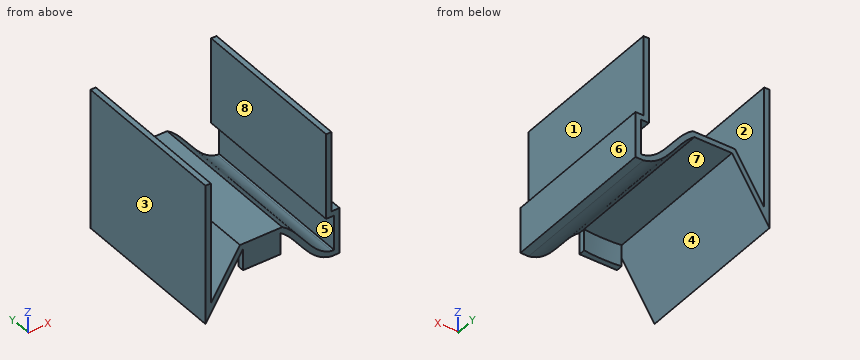
from build123d import *

# Parameters (mm, degrees)
BOSS_EXTRUDE12_DEPTH = 60
BOSS_EXTRUDE13_DEPTH = 8


with BuildPart() as part:
    # Sketch1 → Boss-Extrude12 (new body)
    with BuildSketch(Plane(origin=(0, 0, 0), x_dir=(1, 0, 0), z_dir=(0, 1, 0))):
        with BuildLine():
            Line((3, 47), (3, 30))
            Line((3, 30), (0, 30))
            Line((0, 30), (0, 0))
            Line((0, 0), (-2, 0))
            Line((-2, 0), (-2, 32))
            Line((-2, 32), (1, 32))
            Line((1, 32), (1, 45))
            Line((1, 45), (0.176102142, 45))
            add(Edge.make_bspline(
                [(-18.386432119, 28), (-18.281589374, 28.071011485), (-18.076006872, 28.210643772), (-17.632017964, 28.509033814), (-16.788752159, 29.127765228), (-15.266101597, 30.436706514), (-13.281769764, 32.578807621), (-11.116323446, 35.322397153), (-8.327983452, 38.971629637), (-4.796332276, 42.989291988), (-1.605396872, 44.667429051), (0.176102142, 45)],
                knots=[0.007315744, 0.007315744, 0.007315744, 0.007315744, 0.023228008, 0.039140272, 0.0709648, 0.134613856, 0.261911967, 0.389210078, 0.516508189, 0.771104411, 1.025700634, 1.025700634, 1.025700634, 1.025700634], degree=3))
            Line((-18.386432119, 28), (-34.105031298, 28))
            Line((-34.105031298, 28), (-45, 45.32952773))
            Line((-45, 45.32952773), (-45, 0))
            Line((-45, 0), (-47, 0))
            Line((-47, 0), (-47, 52.268387809))
            Line((-47, 52.268387809), (-33, 30))
            Line((-33, 30), (-19, 30))
            add(Edge.make_bspline(
                [(0, 47), (-8.735842334, 45.522262704), (-12.411198706, 34.462689008), (-19, 30)],
                knots=[0, 0, 0, 0, 1, 1, 1, 1], degree=3))
            Line((0, 47), (3, 47))
        make_face()
    extrude(amount=BOSS_EXTRUDE12_DEPTH)

    # Sketch2 → Boss-Extrude13 (add)
    with BuildSketch(Plane(origin=(0, 0, -30), x_dir=(-1, 0, 0), z_dir=(0, 0, -1))):
        with BuildLine():
            Line((33, 0), (19, 0))
            Line((19, 0), (19, 2.423963318))
            ThreePointArc((19, 2.423963318), (26, 2), (33, 2.423963318))
            Line((33, 2.423963318), (33, 0))
        make_face()
    extrude(amount=BOSS_EXTRUDE13_DEPTH)


solid = part.part
Check sheet for the modelled part. Datum: model origin and axes. Units: mm. Face numbers are marked on the shaded views. A direction names the side the tool comes from. Round coordinates to 2 decimals unless told otherwise and drop trailing zeros. Order: outer loops, then holes, each group sorted by start corner. A loop starts at its lowest first (then second) coordinate and runs counter-clockwise, first axis right, second up.
Q1. Cross-section at C-C, the plane x = -21.5. Enter the section's corners in (y, z), plus the area to 3 significant figures.
Filled sheet:
outline: (0, -38) - (2.17, -38) - (2.17, -30) - (60, -30) - (60, -28) - (0, -28) - close
area: 137 mm2
Q2. Draft check along X on the marked faces 1, 2, 3 and 4. Enter one of: pulls with the +X half, pulls with the -X half, needs draft (parallel to the pull), parting line crosses it, or undercut.
Filled sheet:
face 1: pulls with the +X half
face 2: undercut
face 3: pulls with the -X half
face 4: undercut
Q3. Set-up check for the marked faces 5, 6, 7 and 8: record each of +Z, -Z, +X, -X, +Y, -Y from which the full face is reachable in a straight line by a thin tool's end or side.
Filled sheet:
face 5: +Y, -Y
face 6: +Z, -Z, +X, +Y, -Y
face 7: -Z, +Y
face 8: +Z, +Y, -Y
Q4. Cross-section at B-B, the plane x = -28.5. Enter the section's corners in (y, z), plus the area to 3 significant figures.
Filled sheet:
outline: (0, -38) - (2.05, -38) - (2.05, -30) - (60, -30) - (60, -28) - (0, -28) - close
area: 136 mm2
Q5. Depth check by flat-ended pin: P1, Ø0.9, axis at x = 0.5, y = 25.5, coming from the +Z side; P2, Ø6, axis at x = -26, y = 22, coming from the -Z side; P3, Ø15, axis at y = 42.5, z = -10, coming from the +X side. Enter the tip coordinate at first touch or a pass-through.
Filled sheet:
P1: stops at z = -30
P2: stops at z = -30
P3: stops at x = 0
Q6. Cross-section at A-A, the plane z = -5. Enter the section's corners in (x, y).
Filled sheet:
outline: (-47, 0) - (-45, 0) - (-45, 60) - (-47, 60) - close; (-2, 0) - (0, 0) - (0, 60) - (-2, 60) - close
Q7. Scan lines: L1, parallel to X at y = 18.5, z = -26; L2, parallel to X at y = 43.5, z = -40; L3, parallel to X at y = 31.5, z = -30.5. Record each from-to range of solid material in increasing order.
Filled sheet:
L1: x = -47 to -45, -2 to 0
L2: x = -47 to -45, -41.65 to -39.29, -10 to -7.37, 1 to 3
L3: x = -47 to -45, -35.68 to -33.31, -18.31 to -15.27, -2 to 3
